Geometry: see drawing. Coordinates: mm, zero at the bounding-box minimum. Give positions to 0.01 mm unless a question says otherwise; leave off trailing zeros. Loops run counter-clockwise (first coordinate to the right, second up) from the corner with the lowest first, then second, coordinate; pieces in that order, holes last. Notation, with made-up numbers: (8, 12) -> (63, 12) arc R14 cw to (63, 17) -> close; hole circle Ø3 at (28.5, 81). An arc over 180 degrees is marked (long way). Return JSON: item names as keys, results as strings. Group by question number.
(1) Cut plane C-C on y = 11.75. Return loops of the section in (x, z).
(2) Ray query, line 1 (Y direction, x = 12, z = 19.75); line 2 (X direction, y = 11.5, z = 16.75); line 3 (Z direction, x = 5, y = 9.5) (1 decimal). Return the intervals inside material, ascending. Write a range as from..to.
(3) Cut plane A-A on z = 17.75. Return loops of the section in (x, y), then the cut area to 3 significant figures.
(4) Pin query (flat end, axial travel): pin 1 (6.5 mm diameter, centred on x = 14.5, z = 19, fed in from +Y). Return the tip coordinate at first contact, or that it passes through.
(5) Cut plane B-B on x = 16.5. Return loops of the section in (y, z) (1 decimal).
(6) Draft query along X for the marked faces 1, 2, 3 and 4. Return one class per face: released by +X, released by -X, zero draft, split by the parting line, or undercut.
(7) Cut plane D-D on z = 21.25. Return loops of the section in (x, y).
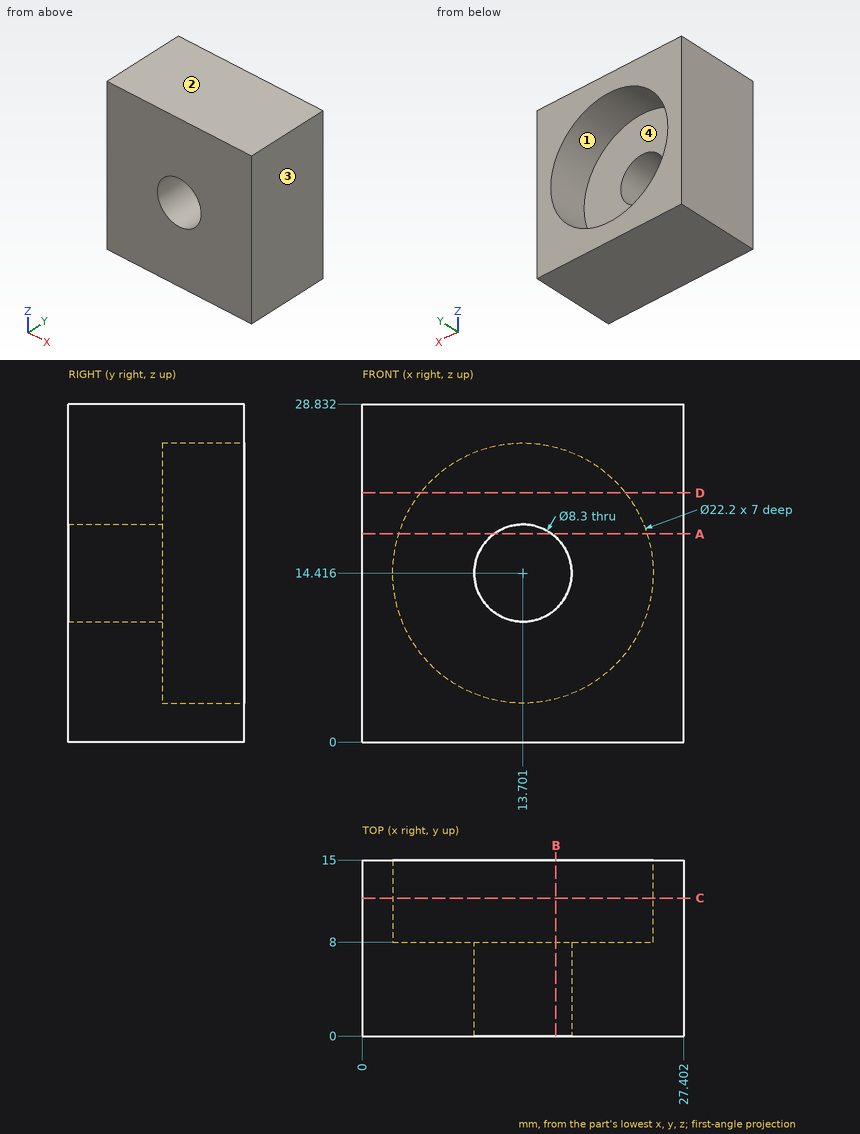
Answers:
{
 "1": {"outline": "(0, 0) -> (27.4, 0) -> (27.4, 28.83) -> (0, 28.83) -> close; hole circle Ø22.2 at (13.7, 14.42)"},
 "2": {"line 1": "0..8", "line 2": "0..2.85, 24.55..27.4", "line 3": "0..7.5, 21.3..28.8"},
 "3": {"outline": "(0, 0) -> (11.23, 0) -> (11.23, 8) -> (3.11, 8) -> (3.11, 15) -> (0, 15) -> close; (16.17, 0) -> (27.4, 0) -> (27.4, 15) -> (24.29, 15) -> (24.29, 8) -> (16.17, 8) -> close", "area": "223 mm²"},
 "4": {"pin 1": "y = 8"},
 "5": {"outline": "(0, 0) -> (15, 0) -> (15, 3.7) -> (8, 3.7) -> (8, 11.4) -> (0, 11.4) -> close; (0, 17.5) -> (8, 17.5) -> (8, 25.2) -> (15, 25.2) -> (15, 28.8) -> (0, 28.8) -> close"},
 "6": {"face 1": "undercut", "face 2": "zero draft", "face 3": "released by +X", "face 4": "undercut"},
 "7": {"outline": "(0, 0) -> (27.4, 0) -> (27.4, 15) -> (22.45, 15) -> (22.45, 8) -> (4.95, 8) -> (4.95, 15) -> (0, 15) -> close"}
}
